Read the model definition and answer for the solid it produces. Units are mm, in the model's axes. Face numbers are marked on the shaded views. A direction names the side the tool comes from. Coordinates: 2 decimals unless noted, no trailing zeros. Order: outer loops, then holes, each group sorted by start corner. A loop starts at its lowest first (then second) coordinate and runs counter-clockwise, first axis right, second up. Notation, with made-up numbers: M 20.5,-4 L 64.5,-4 A13 cw 64.5,21 Z; hole C 74,79 d6. An arc over 180 degrees is marked long. Put each result on its own line as item: value.
from build123d import *

# Parameters (mm, degrees)
SKETCH1_R           = 7.5
SKETCH1_R_2         = 4
BOSS_EXTRUDE1_DEPTH = 24
SKETCH2_R           = 6.35
SKETCH2_R_2         = 4.35
CUT_EXTRUDE1_DEPTH  = 0.5
SKETCH3_R           = 6.35
SKETCH3_R_2         = 4.35
CUT_EXTRUDE2_DEPTH  = 0.5
CHAMFER1_SIZE       = 0.15


with BuildPart() as part:
    # Sketch1 → Boss-Extrude1 (new body)
    with BuildSketch(Plane.XY):
        Circle(SKETCH1_R)
        Circle(SKETCH1_R_2, mode=Mode.SUBTRACT)
    extrude(amount=-BOSS_EXTRUDE1_DEPTH)

    # Sketch2 → Cut-Extrude1 (cut)
    with BuildSketch(Plane.XY):
        Circle(SKETCH2_R)
        Circle(SKETCH2_R_2, mode=Mode.SUBTRACT)
    extrude(amount=-CUT_EXTRUDE1_DEPTH, mode=Mode.SUBTRACT)

    # Sketch3 → Cut-Extrude2 (cut)
    with BuildSketch(Plane(origin=(0, 0, -24), x_dir=(-1, 0, 0), z_dir=(0, 0, -1))):
        Circle(SKETCH3_R)
        Circle(SKETCH3_R_2, mode=Mode.SUBTRACT)
    extrude(amount=-CUT_EXTRUDE2_DEPTH, mode=Mode.SUBTRACT)

    # Groove Sketch → Retaining Ring Groove (revolve, cut)
    with BuildSketch(Plane(origin=(10.524041949, 3.020841974, -25.315160673), x_dir=(-0.243952573, -0.070024633, -0.967255754), z_dir=(-0.27590078, 0.961186121, 0))):
        with BuildLine():
            Line((-16.721138463, 23.21299415), (-16.66022558, 23.445135531))
            Line((-16.66022558, 23.445135531), (-17.724206909, 23.724319577))
            Line((-17.724206909, 23.724319577), (-17.785119792, 23.492178196))
            ThreePointArc((-17.785119792, 23.492178196), (-17.773697794, 23.408766243), (-17.706640064, 23.357861658))
            Line((-17.706640064, 23.357861658), (-16.855455, 23.134514422))
            ThreePointArc((-16.855455, 23.134514422), (-16.772043048, 23.14593642), (-16.721138463, 23.21299415))
        make_face()
    revolve(axis=Axis((0, 0, -38.025873123), (0, 0, 1)), mode=Mode.SUBTRACT)

    # Groove Sketch1 → Retaining Ring Groove1 (revolve, cut)
    with BuildSketch(Plane(origin=(10.524041949, 3.020841974, -25.315160673), x_dir=(-0.243952573, -0.070024633, -0.967255754), z_dir=(-0.27590078, 0.961186121, 0))):
        with BuildLine():
            Line((1.269818557, 18.492245746), (1.33073144, 18.724387127))
            Line((1.33073144, 18.724387127), (0.266750111, 19.003571172))
            Line((0.266750111, 19.003571172), (0.205837228, 18.771429791))
            ThreePointArc((0.205837228, 18.771429791), (0.217259227, 18.688017839), (0.284316956, 18.637113254))
            Line((0.284316956, 18.637113254), (1.13550202, 18.413766017))
            ThreePointArc((1.13550202, 18.413766017), (1.218913972, 18.425188016), (1.269818557, 18.492245746))
        make_face()
    revolve(axis=Axis((0, 0, -38.025873123), (0, 0, 1)), mode=Mode.SUBTRACT)

    # Chamfer1
    chamfer1_edges = [part.edges().sort_by_distance(p)[0] for p in [
        (-6.35, 0, -0.5),
        (-4.35, 0, -0.5),
        (6.35, 0, -23.5),
        (-7.5, 0, 0),
        (4.35, 0, -23.5),
        (-7.5, 0, -24),
    ]]
    chamfer(chamfer1_edges, length=CHAMFER1_SIZE)


solid = part.part
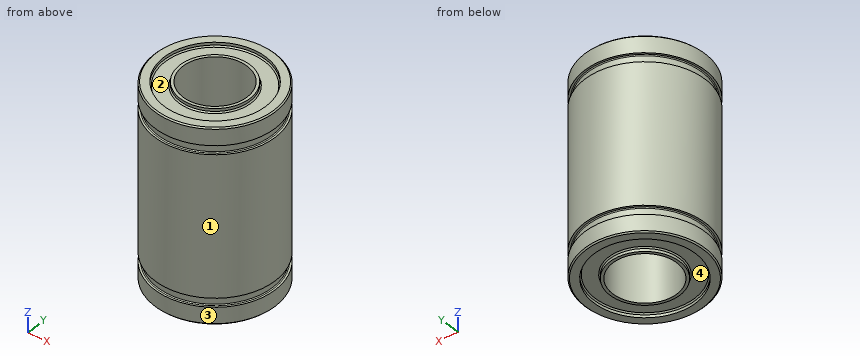
Q1. Consider line 1 along Y through (x, z) = (0, -0.2); line 2 along Y through (x, z) = (0, -14.75); line 3 along Z through (x, y) = (-4, 6). Determine where each line is inside the solid, lowest interval first.
Answers below:
line 1: y = -7.5 to -6.35, -4.35 to -4, 4 to 4.35, 6.35 to 7.5
line 2: y = -7.5 to -4, 4 to 7.5
line 3: z = -24 to -21.84, -20.76 to -3.24, -2.16 to 0
Q2. Find section A-A on z = -22.5. Write down the section's boundary in (x, y).
Answers below:
outline: C 0,0 d15; hole C 0,0 d8
Q3. Given pin 1 (1 mm diameter, centred on x = 0, y = 3, fed in from -Z); pin 2 (3 mm diameter, centred on y = -4.5, z = -21, fed in from -X); pin 3 (5 mm diameter, centred on y = 3.5, z = -8.5, fed in from +X); pin 4 (2 mm diameter, centred on x = 3, z = -10, fed in from -Y), each flat-ended and moving along its own axis, determine where each tip first touches the part or whether it passes through.
Answers below:
pin 1: passes through
pin 2: stops at x = -6.86
pin 3: stops at x = 7.43
pin 4: stops at y = -7.23
Q4. For a pull along X with two mould halves and no side action, classify the marked faces 3 and 4 as +X half, -X half, draft (parallel to the pull), parting line (faces both ways), or undercut.
Answers below:
face 3: parting line
face 4: undercut
Q5. A tool of negligible diameter and unlimited length cuts with its end or side. For the marked faces 1 and 2, from which of +Z, -Z, +X, -X, +Y, -Y can it reach the whole face along a straight path? Write none if from no direction.
Answers below:
face 1: +Z, -Z
face 2: +Z
